Check sheet for the modelled part. Datum: model origin and axes. Units: mm. A direction names the side the tool comes from. Round coordinates to 2 decimals unless told otherwise and drop trailing zeros. Order: outer loops, then holes, each group sorted by start corner. A loop starts at its lowest first (then second) coordinate and runs counter-clockwise, first axis right, second up. Notation, with made-up numbers: (-28.75, 3) -> (26.25, 3) arc R12 ccw to (26.25, 11) -> close; hole circle Ø4 at (-32.75, 5.5). An arc over 180 degrees is marked (long way). Answer in a Markdown table with one row per item.
from build123d import *

# Parameters (mm, degrees)
SKETCH1_W           = 35
SKETCH1_H           = 35
BOSS_EXTRUDE1_DEPTH = 28
CUT_EXTRUDE1_DEPTH  = 57.868268832
CUT_EXTRUDE2_REACH  = 56.215
SKETCH3_W           = 23
SKETCH3_H           = 33.717030155
CUT_EXTRUDE3_DEPTH  = 4.5
CUT_EXTRUDE4_DEPTH  = 4.5
SKETCH6_W           = 1
SKETCH6_H           = 5.8
BOSS_EXTRUDE2_DEPTH = 1
SKETCH7_W           = 5.8
SKETCH7_H           = 1
BOSS_EXTRUDE3_DEPTH = 1


with BuildPart() as part:
    # Sketch1 → Boss-Extrude1 (new body)
    with BuildSketch(Plane.XY):
        with Locations((17.5, 17.5)):
            Rectangle(SKETCH1_W, SKETCH1_H)
    extrude(amount=BOSS_EXTRUDE1_DEPTH)

    # Sketch2 → Cut-Extrude1 (cut, through all)
    with BuildSketch(Plane.XY.offset(28)):
        Polygon((6.5, 37.082021278), (6.5, 33), (33, 6.5), (39.701272532, 6.5), (39.701272532, 37.082021278), align=None)
    extrude(amount=-CUT_EXTRUDE1_DEPTH, mode=Mode.SUBTRACT)

    # Cut-Extrude2: up to this face of the body (flat: up to its plane)
    cut_extrude2_end = Plane(part.part.faces().sort_by_distance((35, 3.25, 14))[0])
    # Sketch3 → Cut-Extrude2 (cut, up to the picked face)
    with BuildSketch(Plane.ZY.offset(-4.5), mode=Mode.PRIVATE) as cut_extrude2_sk1:
        with Locations((14, 21.358515078)):
            Rectangle(SKETCH3_W, SKETCH3_H)
    cut_extrude2_tool1 = split(extrude(cut_extrude2_sk1.sketch, amount=-CUT_EXTRUDE2_REACH, mode=Mode.PRIVATE), bisect_by=cut_extrude2_end, keep=Keep.BOTH, mode=Mode.PRIVATE)
    add(cut_extrude2_tool1.solids().sort_by(Axis((4.5, 21.358515, 14), (1, 0, 0)))[0], mode=Mode.SUBTRACT)

    # Sketch4 → Cut-Extrude3 (cut)
    with BuildSketch(Plane(origin=(4.5, 0, 0), x_dir=(0, 0, -1), z_dir=(1, 0, 0))):
        with BuildLine():
            Line((-10.5, 23.5), (-10.5, 12))
            ThreePointArc((-10.5, 12), (-14, 8.5), (-17.5, 12))
            Line((-17.5, 12), (-17.5, 23.5))
            ThreePointArc((-17.5, 23.5), (-14, 27), (-10.5, 23.5))
        make_face()
    extrude(amount=-CUT_EXTRUDE3_DEPTH, mode=Mode.SUBTRACT)

    # Sketch5 → Cut-Extrude4 (cut)
    with BuildSketch(Plane(origin=(0, 4.5, 0), x_dir=(1, 0, 0), z_dir=(0, 1, 0))):
        with BuildLine():
            Line((23.5, -17.5), (12, -17.5))
            ThreePointArc((12, -17.5), (8.5, -14), (12, -10.5))
            Line((12, -10.5), (23.5, -10.5))
            ThreePointArc((23.5, -10.5), (27, -14), (23.5, -17.5))
        make_face()
    extrude(amount=-CUT_EXTRUDE4_DEPTH, mode=Mode.SUBTRACT)

    # Sketch6 → Boss-Extrude2 (add)
    with BuildSketch(Plane.XZ):
        with Locations((33.5, 14)):
            Rectangle(SKETCH6_W, SKETCH6_H)
    extrude(amount=BOSS_EXTRUDE2_DEPTH)

    # Sketch7 → Boss-Extrude3 (add)
    with BuildSketch(Plane.ZY):
        with Locations((14, 33.5)):
            Rectangle(SKETCH7_W, SKETCH7_H)
    extrude(amount=BOSS_EXTRUDE3_DEPTH)


solid = part.part
Item 1: Mould release check, pull along Z, two halves, no side actions. Record for faces 1 (the flat face through (13, 14, 0)), 2 (the flat face through (2, 18, 17.5)), 3 (the flat face through (19.6, 19.9, 26.8)): pulls with the +Z half, pulls with the -Z half, needs draft (parallel to the pull), parting line crosses it, or undercut.
Result sheet:
| item | result |
|---|---|
| face 1 | pulls with the -Z half |
| face 2 | undercut |
| face 3 | needs draft |
Item 2: Set-up check for faces 4 (the flat face through (-0.5, 33, 14)), 5 (the cylindrical face through (8.5, 2.3, 14.1)), 6 (the cylindrical face through (2, 27, 14)), 7 (the flat face through (6.5, 34, 27)), 8 (the flat face through (4.5, 20, 9)): record each of +Z, -Z, +X, -X, +Y, -Y from which the full face is reachable in a straight line by a thin tool's end or side.
Result sheet:
| item | result |
|---|---|
| face 4 | +Z, -Z, -X, -Y |
| face 5 | +Y, -Y |
| face 6 | +X, -X |
| face 7 | +Z, -Z, +X, +Y |
| face 8 | +X, +Y |
Item 3: Scan lines: line 1 (Z direction, x = 17.5, y = 7.5); line 2 (X direction, y = 19.5, z = 19.25). Record each from-to range of solid material in increasing order. Write a range as [from, to].
Result sheet:
| item | result |
|---|---|
| line 1 | z = [0, 2.5], [25.5, 28] |
| line 2 | x = [0, 4.5] |
Item 4: Cross-section at A-A (x = 18). Record the boundary of the cut face in (y, z), and give its area (4 significant figures).
Result sheet:
| item | result |
|---|---|
| outline | (0, 0) -> (21.5, 0) -> (21.5, 2.5) -> (4.5, 2.5) -> (4.5, 10.5) -> (0, 10.5) -> close; (0, 17.5) -> (4.5, 17.5) -> (4.5, 25.5) -> (21.5, 25.5) -> (21.5, 28) -> (0, 28) -> close |
| area | 179.5 mm^2 |
Item 5: Cross-section at C-C (z = 1.5). Record the boundary of the cut face in (x, y).
Result sheet:
| item | result |
|---|---|
| outline | (0, 0) -> (35, 0) -> (35, 6.5) -> (33, 6.5) -> (6.5, 33) -> (6.5, 35) -> (0, 35) -> close |
Item 6: Depth check by flat-ended pin: P1, Ø7, axis at x = 13.5, z = 19.5, coming from the +Y side; P2, Ø4, axis at y = 14.5, z = 11, coming from the +X side; P3, Ø8.5, axis at y = 12, z = 19.5, coming from the -X side. Enter the tip coordinate at first touch or a pass-through.
Result sheet:
| item | result |
|---|---|
| P1 | stops at y = 4.5 |
| P2 | stops at x = 4.5 |
| P3 | stops at x = 0 |
Item 7: Cross-section at B-B (y = 3). Record the boundary of the cut face in (x, z), and give its area (3 significant figures).
Result sheet:
| item | result |
|---|---|
| outline | (0, 0) -> (35, 0) -> (35, 28) -> (0, 28) -> close; hole (12, 10.5) -> (23.5, 10.5) arc R3.5 ccw to (23.5, 17.5) -> (12, 17.5) arc R3.5 ccw to start |
| area | 861 mm^2 |
